The drawing under review shows one solid part. Ordinate dimensions are in mm from its lowest x, y, z. A direction names the side the tool comes from. Round coordinates to 2 decimals unless told otherwise and drop trailing zeros. Order: outer loops, then holes, each group sorted by start corner. A loop starts at its lowest first (then second) coordinate and runs counter-clockwise, first axis right, second up.
1) Consider section D-D (y = 15.25). Give the boundary of the cut face in (x, z).
2) To check wall thickness, follow L1, parallel to Z at x = 71.5, y = 3.25; L2, parallel to Y at x = 62, z = 10 (1 decimal); L3, parallel to Y at x = 72, z = 9.5 (1 decimal). State the ranges of each line that lie inside material, in increasing order.
3) Clearance check with flat-ended pins moving along their axes: P1, Ø4, axis at x = 33.5, z = 8, coming from the -Y side; P2, Ø2, axis at x = 43, z = 6.5, coming from the +Y side. State where each tip first meets the part, or that it passes through.
4) Consider section C-C (y = 6). Give the boundary of the cut face in (x, z), then the cut area to 3 significant figures.
5) Consider section A-A (z = 12.5). Give the boundary of the cut face in (x, y).
6) Mouldability with a two-part tool opening along Z and no side actions: class the marked faces 4, 5, 6 and 7 as pulls with the +Z half, pulls with the -Z half, needs draft (parallel to the pull), parting line crosses it, or undercut.
7) Machinability: for the marked faces 1, 2 and 3, which of the approach directions +Z, -Z, +X, -X, +Y, -Y give a long, thin tool a straight path to every point of the face, cutting with its end or side? Answer none if there is none.
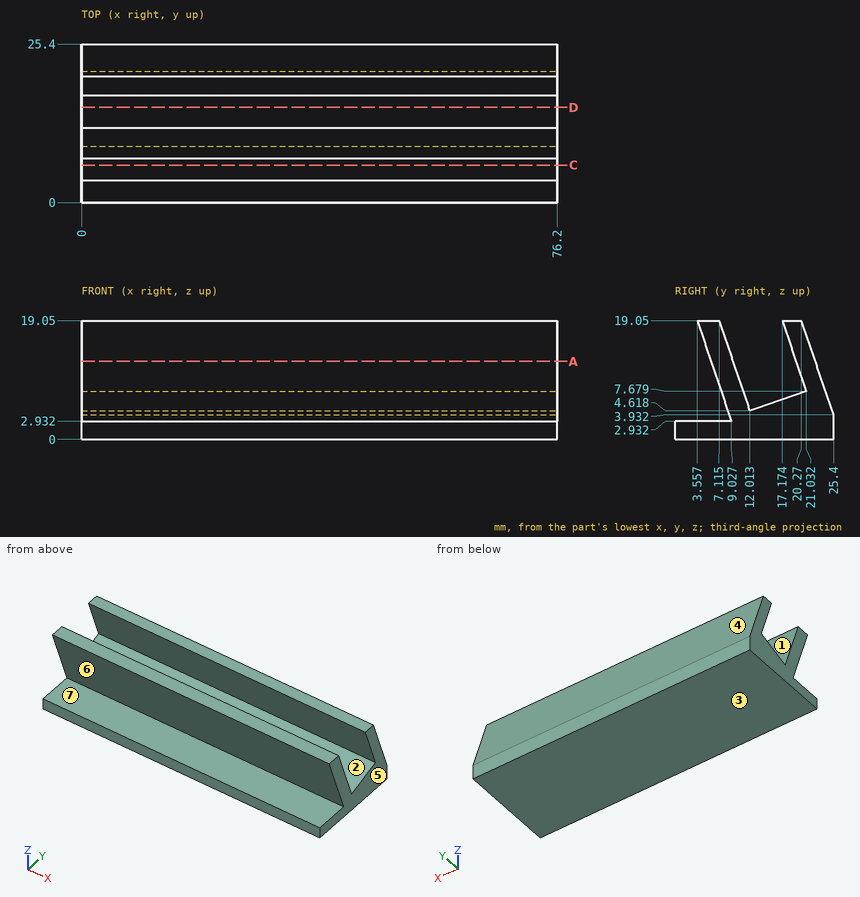
Answer below:
1. outline: (0, 0) - (76.2, 0) - (76.2, 5.72) - (0, 5.72) - close
2. L1: z = 0 to 2.93
2. L2: y = 6.6 to 10.2, 20.2 to 23.3
2. L3: y = 6.8 to 10.4, 20.4 to 23.5
3. P1: stops at y = 6.63
3. P2: stops at y = 24.87
4. outline: (0, 0) - (76.2, 0) - (76.2, 2.93) - (0, 2.93) - close; (0, 11.85) - (76.2, 11.85) - (76.2, 19.05) - (0, 19.05) - close
4. area: 772 mm2
5. outline: (0, 5.78) - (76.2, 5.78) - (76.2, 9.34) - (0, 9.34) - close; (0, 19.4) - (76.2, 19.4) - (76.2, 22.49) - (0, 22.49) - close
6. face 4: pulls with the +Z half
6. face 5: needs draft
6. face 6: undercut
6. face 7: undercut
7. face 1: +Z, +X, -X
7. face 2: +X, -X
7. face 3: -Z, +X, -X, +Y, -Y
